```python
from build123d import *

# Parameters (mm, degrees)
BOSS_EXTRU_1_DEPTH           = 20
ESQUISSE2_R                  = 2
ENL_V_MAT_EXTRU_1_DEPTH      = 35.641016151
ESQUISSE3_R                  = 2
ENL_V_MAT_EXTRU_2_DEPTH      = 35.641016151
ENL_V_MAT_EXTRU_3_DEPTH      = 5
ENL_V_MAT_EXTRU_3_DEPTH_BACK = 5
ESQUISSE6_R                  = 5
ENL_V_MAT_EXTRU_4_DEPTH      = 6
ENL_V_MAT_EXTRU_4_DEPTH_BACK = 5
ESQUISSE9_R                  = 5


with BuildPart() as part:
    # Esquisse1 → Boss.-Extru.1 (new body)
    with BuildSketch(Plane.XY):
        Polygon((0, 0), (-20, 0), (0, -20), align=None)
    extrude(amount=BOSS_EXTRU_1_DEPTH)

    # Esquisse2 → Enlèv. mat.-Extru.1 (cut, through all)
    with BuildSketch(Plane(origin=(0, 0, 0), x_dir=(1, 0, 0), z_dir=(0, 1, 0))):
        with Locations(Location((-10, -10, 0), (0, 0, 180))):
            Circle(ESQUISSE2_R)
    extrude(amount=-ENL_V_MAT_EXTRU_1_DEPTH, mode=Mode.SUBTRACT)

    # Esquisse3 → Enlèv. mat.-Extru.2 (cut, through all)
    with BuildSketch(Plane(origin=(0, 0, 0), x_dir=(0, 0, -1), z_dir=(1, 0, 0))):
        with Locations((-10, -10)):
            Circle(ESQUISSE3_R)
    extrude(amount=-ENL_V_MAT_EXTRU_2_DEPTH, mode=Mode.SUBTRACT)

    # Esquisse6 → Enlèv. mat.-Extru.3 (cut, two sides: drawn at the far end of the back side and taken through both)
    with BuildSketch(Plane(origin=(0, -10, 0), x_dir=(1, 0, 0), z_dir=(0, 1, 0)).offset(-ENL_V_MAT_EXTRU_3_DEPTH_BACK)):
        with Locations((-10.004008989, -9.994708572)):
            Circle(ESQUISSE6_R)
    extrude(amount=ENL_V_MAT_EXTRU_3_DEPTH + ENL_V_MAT_EXTRU_3_DEPTH_BACK, mode=Mode.SUBTRACT)

    # Esquisse9 → Enlèv. mat.-Extru.4 (cut, two sides: drawn at the far end of the back side and taken through both)
    with BuildSketch(Plane(origin=(-10, 0, 0), x_dir=(0, 0, -1), z_dir=(1, 0, 0)).offset(-ENL_V_MAT_EXTRU_4_DEPTH_BACK)):
        with Locations(Location((-9.969497879, -10.041855886, 0), (0, 0, 208.496581374))):
            Circle(ESQUISSE9_R)
    extrude(amount=ENL_V_MAT_EXTRU_4_DEPTH + ENL_V_MAT_EXTRU_4_DEPTH_BACK, mode=Mode.SUBTRACT)


solid = part.part
```
The model under review builds one solid part; all positions refer to its coordinate system, in mm. A direction names the side the tool comes from. Coordinates: 2 decimals unless noted, no trailing zeros. Write each loop counter-clockwise with the first axis right and the second up, starting at its lowest first coordinate (ties: lowest second). Pieces come first, ordered by that corner, then holes. Notation, with made-up numbers: (28, 50.25) - (49, 50.25) arc R25 ccw to (49, 86.25) - close; hole circle Ø11 at (-13, -16). An arc over 180 degrees is marked (long way). Answer in a Markdown table with one row per item. Add a question column.
Q1. Consider section B-B on x = -10. Give the boundary of the cut face in (y, z).
Q2. Clearance check with flat-ended pins moving along their axes: pin 1 (1 mm diameter, centred on y = -4, z = 14, fed in from -X); pin 2 (12 mm diameter, centred on x = -16, y = -18, fed in from +Z); pin 3 (8 mm diameter, centred on x = -18, z = 13.5, fed in from -Y); pin 4 (5 mm diameter, centred on x = -9, z = 10, fed in from -Y). State where each tip first meets the part, or that it passes through.
Q3. Consider section D-D on y = -2.75. Give the boundary of the cut face in (x, z), then the cut area to 3 significant figures.
Q4. Consider section C-C on z = 11.5. Give the boundary of the cut face in (x, y).
Q5. Consider section A-A on y = -10. Give the boundary of the cut face in (x, z).
Q6. Draft analysis for pull direction Y (two halves, no side actions). For faces 4 (the face through (-12, -8, 5)), 5 (the face through (-6, -5, 0)), 6 (the face through (-2, -8, 10)), state which applies: +Y half, -Y half, draft (parallel to the pull), parting line (faces both ways), or undercut.
Q7. For faces 1 (the face through (-10.07, -5, 12.15)), 2 (the face through (-6, -7, 6)), 3 (the face through (-6, -5, 20)), list the 3-axis set-ups (+Z, -Z, +X, -X, +Y, -Y) from which the entire face can be reached by the end or side of a thin tool; tool diameter is ignored.
Q8. To check wall thickness, follow line 1 along X through (y, z) = (-8.25, 8); line 2 along Z through (x, y) = (-9.5, -2); line 3 along Y through (x, z) = (-1.15, 10). State the ranges of each line that lie inside material, in increasing order. Write a range as from..to.
Answers below:
| question | item | result |
|---|---|---|
| 1 | outline | (-10, 0) - (0, 0) - (0, 8) - (-5, 8) - (-5, 4.99) - (-9.54, 4.99) arc R5 cw to (-10, 4.97) - close; (-10, 14.99) - (-5, 14.99) - (-5, 12) - (0, 12) - (0, 20) - (-10, 20) - close |
| 2 | pin 1 | x = -16.5 |
| 2 | pin 2 | through |
| 2 | pin 3 | y = -6 |
| 2 | pin 4 | y = -5 |
| 3 | outline | (-17.25, 0) - (0, 0) - (0, 20) - (-17.25, 20) - close; hole circle Ø4 at (-10, 10) |
| 3 | area | 332 mm² |
| 4 | outline | (-20, 0) - (-14.77, -5.23) - (-14.77, -5) - (-11.32, -5) - (-11.32, 0) - close; (-8.68, -5) - (-5.24, -5) - (-5.24, -5.28) - (-4, -5.28) - (-4, -8.68) - (0, -8.68) - (0, 0) - (-8.68, 0) - close; (-5.2, -14.8) - (0, -20) - (0, -11.32) - (-4, -11.32) - (-4, -14.8) - close |
| 5 | outline | (-10, 0) - (0, 0) - (0, 8) - (-4, 8) - (-4, 4.97) - (-10, 4.97) - close; (-10, 14.99) arc R5 cw to (-9.5, 14.97) - (-4, 14.97) - (-4, 12) - (0, 12) - (0, 20) - (-10, 20) - close |
| 6 | face 4 | -Y half |
| 6 | face 5 | draft |
| 6 | face 6 | undercut |
| 7 | face 1 | -Y |
| 7 | face 2 | -X |
| 7 | face 3 | +Z, +X, -X, +Y, -Y |
| 8 | line 1 | -4..0 |
| 8 | line 2 | 0..8.06, 11.94..20 |
| 8 | line 3 | -18.85..-12, -8..0 |
